from build123d import *

# Parameters (mm, degrees)
SKETCH1_W               = 139.7
SKETCH1_H               = 76.2
BOSS_EXTRUDE1_DEPTH     = 38.1
CUT_EXTRUDE1_DEPTH      = 89.217019333
CUT_EXTRUDE1_DEPTH_BACK = 31.75
SKETCH3_R               = 2.032
CUT_EXTRUDE2_DEPTH      = 89.217019333
SKETCH4_W               = 52.07
SKETCH4_H               = 25.4
CUT_EXTRUDE3_DEPTH      = 10.414
SKETCH7_W               = 57.15
SKETCH7_H               = 12.7
BOSS_EXTRUDE2_DEPTH     = 25.4
SKETCH8_W               = 57.15
SKETCH8_H               = 50.8
BOSS_EXTRUDE3_DEPTH     = 12.7
SKETCH5_R               = 2.286
SKETCH5_R_2             = 2.54
CUT_EXTRUDE4_DEPTH      = 109.570070904
CUT_EXTRUDE5_DEPTH      = 14.986
CUT_EXTRUDE6_DEPTH      = 7.112
SKETCH10_R              = 2.159
CUT_EXTRUDE7_DEPTH      = 139.84509874
SKETCH11_W              = 52.07
SKETCH11_H              = 6.35
BOSS_EXTRUDE4_DEPTH     = 25.4


with BuildPart() as part:
    # Sketch1 → Boss-Extrude1 (new body)
    with BuildSketch(Plane(origin=(0, 0, 0), x_dir=(1, 0, 0), z_dir=(0, 1, 0))):
        Rectangle(SKETCH1_W, SKETCH1_H)
    extrude(amount=-BOSS_EXTRUDE1_DEPTH)

    # Sketch2 → Cut-Extrude1 (cut, two sides: drawn at the far end of the back side and taken through both)
    with BuildSketch(Plane.XZ.offset(38.1).offset(-CUT_EXTRUDE1_DEPTH_BACK)):
        Polygon((387.819108191, 26.67), (69.85, 26.67), (7.62, 26.67), (7.62, 0), (-58.42, 0), (-58.42, -38.1), (-58.42, -356.069108191), (355.598009183, -838.77657978), (801.837117374, -456.037471588), align=None)
    extrude(amount=CUT_EXTRUDE1_DEPTH + CUT_EXTRUDE1_DEPTH_BACK, mode=Mode.SUBTRACT)

    # Sketch3 → Cut-Extrude2 (cut, through all)
    with BuildSketch(Plane.XZ.offset(38.1)):
        with Locations(Location((-53.34, 21.59, 0), (0, 0, 270))):
            Circle(SKETCH3_R)
    extrude(amount=-CUT_EXTRUDE2_DEPTH, mode=Mode.SUBTRACT)

    # Sketch4 → Cut-Extrude3 (cut)
    with BuildSketch(Plane(origin=(0, 0, 0), x_dir=(-1, 0, 0), z_dir=(0, 0, -1))):
        with Locations((32.385, -19.05)):
            Rectangle(SKETCH4_W, SKETCH4_H)
    extrude(amount=-CUT_EXTRUDE3_DEPTH, mode=Mode.SUBTRACT)

    # Sketch7 → Boss-Extrude2 (add)
    with BuildSketch(Plane.XY.offset(38.1)):
        with Locations((-41.275, -6.35)):
            Rectangle(SKETCH7_W, SKETCH7_H)
    extrude(amount=BOSS_EXTRUDE2_DEPTH)

    # Sketch8 → Boss-Extrude3 (add)
    with BuildSketch(Plane.XY.offset(63.5)):
        with Locations((-41.275, -25.4)):
            Rectangle(SKETCH8_W, SKETCH8_H)
    extrude(amount=BOSS_EXTRUDE3_DEPTH)

    # Sketch5 → Cut-Extrude4 (cut, through all)
    with BuildSketch(Plane(origin=(0, 0, 10.414), x_dir=(-1, 0, 0), z_dir=(0, 0, -1))):
        with Locations((46.99, -19.05)):
            Circle(SKETCH5_R)
        with Locations((34.29, -19.05)):
            Circle(SKETCH5_R_2)
        with Locations((21.59, -19.05)):
            Circle(SKETCH5_R_2)
    extrude(amount=-CUT_EXTRUDE4_DEPTH, mode=Mode.SUBTRACT)

    # Sketch6 → Cut-Extrude5 (cut)
    with BuildSketch(Plane(origin=(0, 0, 10.414), x_dir=(-1, 0, 0), z_dir=(0, 0, -1))):
        with BuildLine():
            Line((27.051, -18.288), (26.612524863, -18.288))
            ThreePointArc((26.612524863, -18.288), (16.51, -19.05), (26.612524863, -19.812))
            Line((26.612524863, -19.812), (27.051, -19.812))
            Line((27.051, -19.812), (27.051, -21.082))
            Line((27.051, -21.082), (28.829, -21.082))
            Line((28.829, -21.082), (28.829, -19.812))
            Line((28.829, -19.812), (29.267475137, -19.812))
            ThreePointArc((29.267475137, -19.812), (39.37, -19.05), (29.267475137, -18.288))
            Line((29.267475137, -18.288), (28.829, -18.288))
            Line((28.829, -18.288), (28.829, -17.018))
            Line((28.829, -17.018), (27.051, -17.018))
            Line((27.051, -17.018), (27.051, -18.288))
        make_face()
    extrude(amount=-CUT_EXTRUDE5_DEPTH, mode=Mode.SUBTRACT)

    # Sketch9 → Cut-Extrude6 (cut)
    with BuildSketch(Plane(origin=(0, 0, 63.5), x_dir=(-1, 0, 0), z_dir=(0, 0, -1))):
        Polygon((42.323188216, -16.865376771), (42.323188216, -46.634623229), (44.704, -49.276), (49.276, -49.276), (51.656811784, -46.634623229), (51.656811784, -16.865376771), (49.276, -14.224), (44.704, -14.224), align=None)
    extrude(amount=-CUT_EXTRUDE6_DEPTH, mode=Mode.SUBTRACT)

    # Sketch10 → Cut-Extrude7 (cut, through all)
    with BuildSketch(Plane(origin=(0, 0, 70.612), x_dir=(-1, 0, 0), z_dir=(0, 0, -1))):
        with Locations((46.99, -19.05)):
            Circle(SKETCH10_R)
        with Locations((46.99, -31.75)):
            Circle(SKETCH10_R)
        with Locations((46.99, -44.45)):
            Circle(SKETCH10_R)
    extrude(amount=-CUT_EXTRUDE7_DEPTH, mode=Mode.SUBTRACT)

    # Sketch11 → Boss-Extrude4 (add)
    with BuildSketch(Plane(origin=(0, 0, 0), x_dir=(-1, 0, 0), z_dir=(0, 0, -1))):
        with Locations((32.385, -34.925)):
            Rectangle(SKETCH11_W, SKETCH11_H)
    extrude(amount=BOSS_EXTRUDE4_DEPTH)


solid = part.part
Here's how the part is built. I have some questions about the finished solid (model axes, mm). A direction names the side the tool comes from. Round coordinates to 2 decimals unless told otherwise and drop trailing zeros. Loops run counter-clockwise (first coordinate to the right, second up) from the corner with the lowest first, then second, coordinate; pieces in that order, holes last.
1. If we section it at A-A on x = -34.29: Write out the boundary of the cut face in (y, z), plus the area to 3 significant figures.
Answer list:
outline: (-50.8, 63.5) - (-21.59, 63.5) - (-21.59, 76.2) - (-50.8, 76.2) - close; (-38.1, -25.4) - (-31.75, -25.4) - (-31.75, 10.41) - (-24.13, 10.41) - (-24.13, 25.4) - (-21.59, 25.4) - (-21.59, 38.1) - (-38.1, 38.1) - close; (-16.51, 25.4) - (-13.97, 25.4) - (-13.97, 10.41) - (-6.35, 10.41) - (-6.35, -38.1) - (0, -38.1) - (0, 76.2) - (-16.51, 76.2) - (-16.51, 63.5) - (-12.7, 63.5) - (-12.7, 38.1) - (-16.51, 38.1) - close
area: 2,280 mm2
2. Which directions (+Z, -Z, +X, -X, +Y, -Y) give clear straight access to the entire face, cutting with the end or side of a thin tool? Please do faces 1 (the face through (7.62, -22, 14)), 2 (the face through (-42, -12.7, 51)), 3 (the face through (-47, -49.276, 67)).
Answer list:
face 1: -Z, +X, -Y
face 2: +X, -X, -Y
face 3: -Z
3. If we section it at B-B on z = 66.5: Write out the boundary of the cut face in (x, y), plus the area to 3 significant figures.
Answer list:
outline: (-69.85, -50.8) - (-12.7, -50.8) - (-12.7, 0) - (-69.85, 0) - close; hole (-51.66, -46.63) - (-49.28, -49.28) - (-44.7, -49.28) - (-42.32, -46.63) - (-42.32, -16.87) - (-44.7, -14.22) - (-49.28, -14.22) - (-51.66, -16.87) - close; hole circle Ø5.08 at (-34.29, -19.05); hole circle Ø5.08 at (-21.59, -19.05)
area: 2,550 mm2
4. If we section it at C-C on y = -44.45: Write out the boundary of the cut face in (x, z), plus the area to 3 significant figures.
Answer list:
outline: (-69.85, 63.5) - (-51.66, 63.5) - (-51.66, 70.61) - (-49.15, 70.61) - (-49.15, 76.2) - (-69.85, 76.2) - close; (-44.83, 70.61) - (-42.32, 70.61) - (-42.32, 63.5) - (-12.7, 63.5) - (-12.7, 76.2) - (-44.83, 76.2) - close
area: 635 mm2
5. If I drill on line 1 along X through (y, z) = (-19, 14); line 2 along Z through (x, y) = (-27, -31); line 3 along Y through (x, z) = (-46.99, 32), over which ranges is the centre line in solid material (lowest first)?
Answer list:
line 1: x = -69.85 to -49.28, -44.7 to -39.37, -16.51 to 7.62
line 2: z = 10.41 to 38.1, 63.5 to 76.2
line 3: y = -38.1 to -21.34, -16.76 to 0
6. We'd pull the mould along Z, two halves only. Please class faces 4 (the face through (15, -23, 38.1)), 5 (the face through (-6.35, -19, 5)), 6 (the face through (-47, -14.224, 67)), 7 (the face through (-32, -35, -25.4)): +Z half, -Z half, draft (parallel to the pull), parting line (faces both ways), or undercut.
Answer list:
face 4: undercut
face 5: draft
face 6: undercut
face 7: -Z half
7. If we section it at D-D on z = -5: Write out the boundary of the cut face in (x, y).
Answer list:
outline: (-69.85, -38.1) - (-6.35, -38.1) - (-6.35, -31.75) - (-58.42, -31.75) - (-58.42, -6.35) - (69.85, -6.35) - (69.85, 0) - (-69.85, 0) - close
8. For P1, Ø0.9, axis at x = -28, z = 14, coming from the -Y side; P2, Ø8, axis at x = 38, y = -42, coming from the +Z side; P3, Ø1, axis at x = -14.5, z = 32.5, coming from the +Y side; P4, Ø1.5, axis at x = -35.5, y = -26, coming from the -Z side, each with a flat end and sliding along its axis, tell me the tip position at first contact or that it passes through.
Answer list:
P1: stops at y = -38.1
P2: stops at z = 38.1
P3: stops at y = 0
P4: stops at z = 10.41
